The listing builds one solid part. Answer for the finished solid, in the listing's coordinates (mm). Face numbers are marked on the shaded views. A direction names the side the tool comes from. Coordinates: 2 decimals unless noted, no trailing zeros. Order: outer loops, then holes, each group sorted by start corner. A loop starts at its lowest first (then second) coordinate and runs counter-clockwise, first axis right, second up. Notation, with made-up numbers: M 47,-28 L 92,-28 A12 ccw 92,-6 Z; hole C 87,54 d5. An arc over 180 degrees is marked long. One line per item, written item: value. Start each with the question number.
Q1. The part is cut by section A-A on y = -6. Give the vertices of the cut face in (x, z), then the cut area to 3 significant figures.
Q2. Each of these flat-tipped pins is pushed along its axis until it touches: pin 1 Ø5 at (x, y) = (-51, -20) entering from -Z; pin 2 Ø8 at (x, y) = (7.5, -5) entering from -Z; pin 3 Ø5 at (y, z) = (-9.5, 44) entering from -X. Where does it stop, or does it pass through?
Q3. The part is cut by section D-D on z = 10. Give the vertices of the cut face in (x, y), then the cut area to 3 significant figures.
Q4. For the marked faces 1 and 2, determine the directions among +Z, -Z, +X, -X, +Y, -Y from which every point of the face is accessible in a straight line to the end or side of a thin tool.
Q5. Straight lines are drawn through the part: line 1 along Z through (x, y) = (0, -12); line 2 along Y through (x, z) = (-30.5, 15.5); line 3 along X through (y, z) = (-19, 10.5). For each, find the intervals that lie inside material, in ascending order. Write a range as [from, to].
Q6. The part is cut by section B-B on z = 23.5. Give the vertices of the cut face in (x, y), then the cut area to 3 significant figures.
Q7. The part is cut by section C-C on x = 16. Give the vertices of the cut face in (y, z).
Q8. Determine the mould class of the marked faces 3, 4, 5 and 6 for opening direction X: pulls with the +X half, pulls with the -X half, needs draft (parallel to the pull), parting line crosses it, or undercut.
```python
from build123d import *

# Parameters (mm, degrees)
F1_DEPTH = 46
F3_DEPTH = 36
F4_W     = 36
F4_H     = 4
F5_DEPTH = 60
F7_DEPTH = 25
F9_D     = 4.5


with BuildPart() as f1:
    # F0 (on Front) → F1 (new body)
    with BuildSketch(Plane.XZ):
        with BuildLine():
            Line((-55, 0), (55, 0))
            ThreePointArc((55, 0), (0, 55), (-55, 0))
        make_face()
    extrude(amount=F1_DEPTH)

    # F2 (on face) → F3 (cut)
    with BuildSketch(Plane(origin=(0, 0, 0), x_dir=(-1, 0, 0), z_dir=(0, 1, 0))):
        with BuildLine():
            Line((-45, 0), (45, 0))
            ThreePointArc((45, 0), (0, 45), (-45, 0))
        make_face()
    extrude(amount=-F3_DEPTH, mode=Mode.SUBTRACT)

    # F4 (on Right) → F5 (cut, symmetric)
    with BuildSketch(Plane.YZ):
        with Locations((-18, 2)):
            Rectangle(F4_W, F4_H)
    extrude(amount=F5_DEPTH, both=True, mode=Mode.SUBTRACT)

    # F6 (on face) → F7 (cut)
    with BuildSketch(Plane(origin=(0, -36, 0), x_dir=(-1, 0, 0), z_dir=(0, 1, 0))):
        with BuildLine():
            ThreePointArc((0, 7.5), (12.3743686708, 12.6256313292), (17.5, 25))
            ThreePointArc((17.5, 25), (12.3743686708, 37.3743686708), (0, 42.5))
            Line((0, 42.5), (0, 7.5))
        make_face()
        with BuildLine():
            Line((0, 7.5), (0, 42.5))
            ThreePointArc((0, 42.5), (-17.5, 25), (0, 7.5))
        make_face()
    extrude(amount=-F7_DEPTH, mode=Mode.SUBTRACT)

    # F9 (through all)
    with Locations(Plane.XZ.offset(46)):
        with Locations((48.9897948557, 10), (0, 50), (-48.9897948557, 10)):
            Hole(F9_D / 2)


solid = f1.part
```
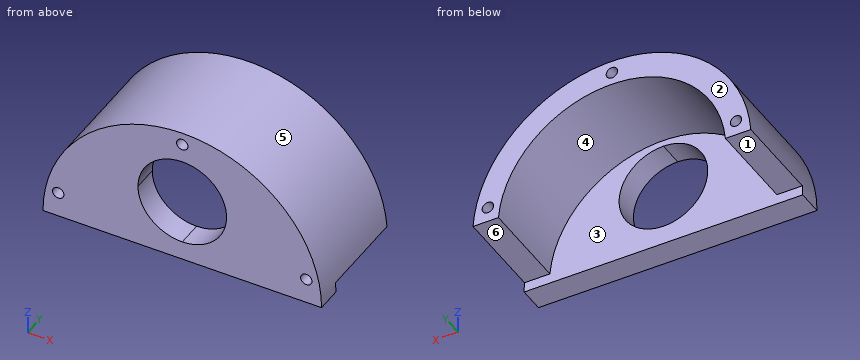
Output:
1. outline: M -54.85,4 L -44.82,4 A45 cw 44.82,4 L 54.85,4 A55 ccw Z; hole C -48.99,10 d4.5; hole C 0,50 d4.5; hole C 48.99,10 d4.5
1. area: 1,440 mm^2
2. pin 1: stops at z = 4
2. pin 2: stops at z = 43.51
2. pin 3: stops at x = -36.09
3. outline: M -54.08,-46 L -51.24,-46 L -51.24,0 L -54.08,0 Z; M -46.74,-46 L -9.01,-46 L -9.01,-36 L -43.87,-36 L -43.87,0 L -46.74,0 Z; M 9.01,-46 L 46.74,-46 L 46.74,0 L 43.87,0 L 43.87,-36 L 9.01,-36 Z; M 51.24,-46 L 54.08,-46 L 54.08,0 L 51.24,0 Z
3. area: 1,220 mm^2
4. face 1: -Z, +X, -X, +Y
4. face 2: +Z, -Z, +X, -X, +Y
5. line 1: z = [45, 47.75], [52.25, 55]
5. line 2: y = [-46, -36]
5. line 3: x = [-53.99, -51.18], [-46.8, -43.76], [43.76, 46.8], [51.18, 53.99]
6. outline: M -49.73,-46 L -17.44,-46 L -17.44,-36 L -38.38,-36 L -38.38,0 L -49.73,0 Z; M 17.44,-46 L 49.73,-46 L 49.73,0 L 38.38,0 L 38.38,-36 L 17.44,-36 Z
6. area: 1,460 mm^2
7. outline: M -46,0 L -36,0 L -36,17.91 L -46,17.91 Z; M -46,32.09 L -36,32.09 L -36,42.06 L 0,42.06 L 0,52.62 L -46,52.62 Z
8. face 3: undercut
8. face 4: undercut
8. face 5: parting line crosses it
8. face 6: needs draft
